For this review, use the dimensioned drawing (mm, ordinates from the lowest corner) and the shaded views. A direction names the side the tool comes from. Coordinates: 2 decimals unless noted, no trailing zeros. Order: outer loops, then holes, each group sorted by start corner. A loop starts at its lowest first (then second) coordinate and runs counter-clockwise, first axis right, second up. Notation, with made-up numbers: M 8.25,47.5 L 38.25,47.5 A18 cw 38.25,62.5 Z; hole C -34,59 d3. An arc over 180 degrees is marked long. Answer in a Markdown table with one row per item.
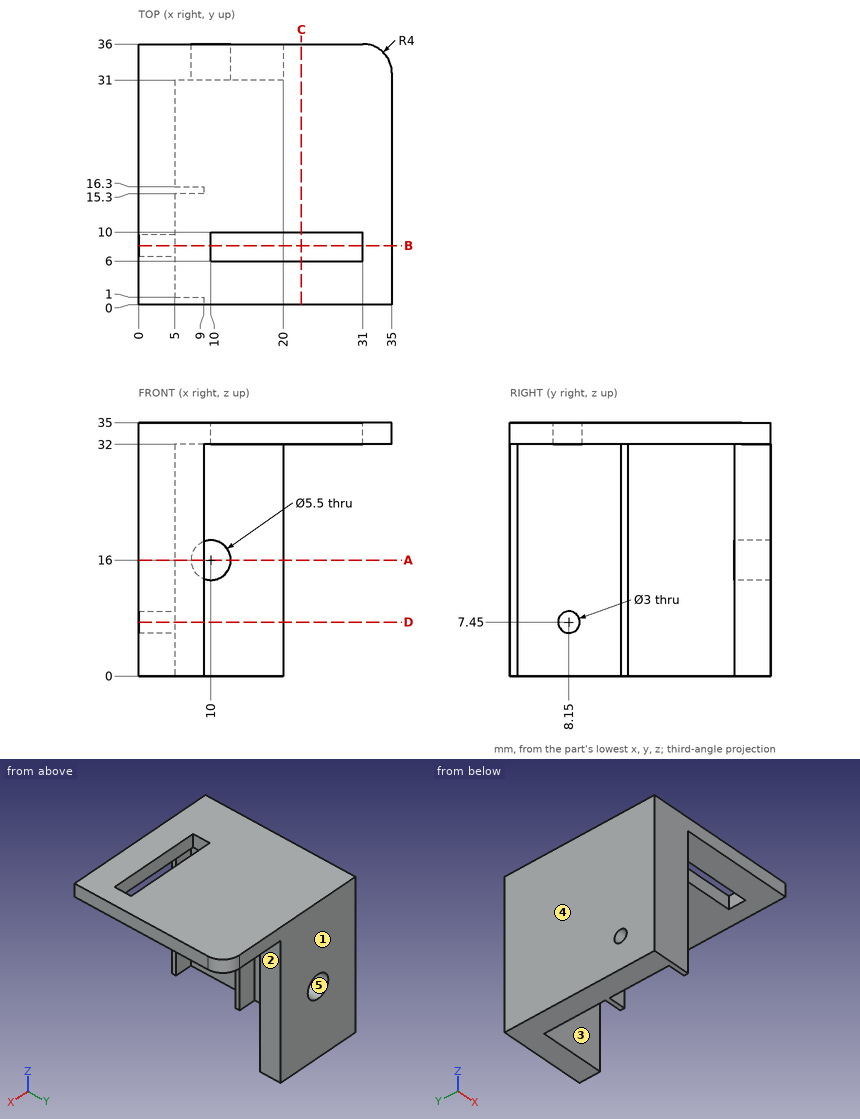
(1) For the marked faces 4 and 5, list the 3-axis set-ups (+Z, -Z, +X, -X, +Y, -Y) from which the entire face can be reached by the end or side of a thin tool; tool diameter is ignored.
Return value:
| item | result |
|---|---|
| face 4 | +Z, -Z, -X, +Y, -Y |
| face 5 | +Y |
(2) For line 1 along Y through (x, z) = (1.75, 7.45); line 2 along Z through (x, y) = (10, 34.55); line 3 along Z through (x, y) = (3.35, 8.15), list the stretches that pass through material, from the lowest coordinate up. Write a range as from..to.
Return value:
| item | result |
|---|---|
| line 1 | y = 0..6.65, 9.65..36 |
| line 2 | z = 0..13.25, 18.75..35 |
| line 3 | z = 0..5.95, 8.95..35 |
(3) Insertion check: pin 1 Ø9 at (x, z) = (10, 16) entering from -Y; pin 2 Ø0.8 at (y, z) = (15.5, 15.5) entering from +X; pin 3 Ø8 at (x, y) = (29.5, 9) entering from -Z; pin 4 Ø5.5 at (y, z) = (33.5, 16.5) entering from +X. Each pin has a flat end and moves straight along its axis. Give the tip position at first contact, or say it passes through.
Return value:
| item | result |
|---|---|
| pin 1 | stops at y = 0 |
| pin 2 | stops at x = 9 |
| pin 3 | stops at z = 32 |
| pin 4 | stops at x = 20 |
(4) Draft analysis for pull direction Y (two halves, no side actions). For the marked faces 1, 2 and 3, state which applies: pulls with the +Y half, pulls with the -Y half, needs draft (parallel to the pull), parting line crosses it, or undercut.
Return value:
| item | result |
|---|---|
| face 1 | pulls with the +Y half |
| face 2 | needs draft |
| face 3 | undercut |
(5) Add section C-C, the plane x = 22.5. Give the boundary of the cut face in (y, z).
Return value:
| item | result |
|---|---|
| outline | M 0,32 L 6,32 L 6,35 L 0,35 Z; M 10,32 L 36,32 L 36,35 L 10,35 Z |
(6) Add section A-A, the plane z = 16. Give the boundary of the cut face in (x, y), and give its area (4 significant figures).
Return value:
| item | result |
|---|---|
| outline | M 0,0 L 9,0 L 9,1 L 5,1 L 5,15.3 L 9,15.3 L 9,16.3 L 5,16.3 L 5,31 L 7.25,31 L 7.25,36 L 0,36 Z; M 12.75,31 L 20,31 L 20,36 L 12.75,36 Z |
| area | 235.5 mm2 |
(7) Add section B-B, the plane y = 8.15. Give the boundary of the cut face in (x, z), and give its area (3 significant figures).
Return value:
| item | result |
|---|---|
| outline | M 0,0 L 5,0 L 5,5.95 L 0,5.95 Z; M 0,8.95 L 5,8.95 L 5,32 L 10,32 L 10,35 L 0,35 Z; M 31,32 L 35,32 L 35,35 L 31,35 Z |
| area | 187 mm2 |
(8) Add section D-D, the plane z = 7.45. Give the boundary of the cut face in (x, y).
Return value:
| item | result |
|---|---|
| outline | M 0,0 L 9,0 L 9,1 L 5,1 L 5,6.65 L 0,6.65 Z; M 0,9.65 L 5,9.65 L 5,15.3 L 9,15.3 L 9,16.3 L 5,16.3 L 5,31 L 20,31 L 20,36 L 0,36 Z |
